```python
from build123d import *

# Parameters (mm, degrees)
ESQUISSE2_R = 0.5


with BuildPart() as part:
    # Balayage1: sweep along a path in Esquisse1
    with BuildLine(Plane.XY) as balayage1_path:
        Line((0, 0), (15, 0))
        ThreePointArc((15, 0), (17.492346414, 3.91220022), (12.893377781, 4.517665927))
        Line((12.893377781, 4.517665927), (11.143330468, 2.432040753))
        ThreePointArc((11.143330468, 2.432040753), (10.136256816, 1.85060651), (8.991054914, 2.052536503))
        Line((8.991054914, 2.052536503), (7.35, 3))
        ThreePointArc((7.35, 3), (6.5, 3.227756814), (5.65, 3))
        Line((5.65, 3), (3.35, 1.672094381))
        ThreePointArc((3.35, 1.672094381), (2.5, 1.444337567), (1.65, 1.672094381))
        Line((1.65, 1.672094381), (0, 2.624722325))
    # Esquisse2 → Balayage1 (sweep)
    with BuildSketch(Plane(origin=(0, 0, 0), x_dir=(0, 0, -1), z_dir=(1, 0, 0))):
        Circle(ESQUISSE2_R)
    sweep(path=balayage1_path.line)


solid = part.part
```
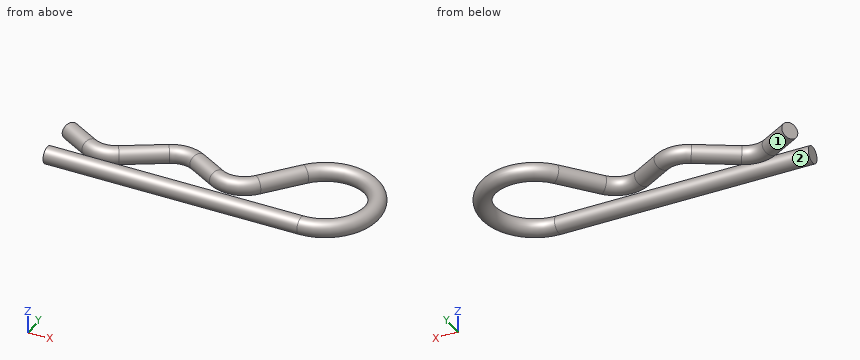
Input: part model. Units: mm. Frame: model coordinates. Face numbers are marked on the shaded views. A direction names the side the tool comes from. Round coordinates to 2 decimals unless told otherwise and drop trailing zeros. Order: outer loops, then holes, each group sorted by start corner. A loop starts at its lowest first (then second) coordinate and runs counter-clockwise, first axis right, second up. Notation, with made-up numbers: (-2.75, 47) - (13.25, 47) arc R24 cw to (13.25, 86) - close; hole circle Ø5 at (3, 84). An arc over 180 degrees is marked (long way). Answer in a Markdown table with one row per item.
Item 1: Line query: line 1 (Z direction, x = 12.5, y = 4); line 2 (Y direction, x = 14.5, z = -0.4); line 3 (Y direction, x = 6, z = 0). Output: solid intervals per line, ascending.
Model answer:
| item | result |
|---|---|
| line 1 | z = -0.5 to 0.5 |
| line 2 | y = -0.3 to 0.3, 5.15 to 5.76 |
| line 3 | y = -0.5 to 0.5, 2.62 to 3.67 |
Item 2: Pin query (flat end, axial travel): pin 1 (0.5 mm diameter, centred on y = 0, z = 0, fed in from -X). Return the tip coordinate at first contact, or that it passes through.
Model answer:
| item | result |
|---|---|
| pin 1 | stops at x = 0 |
Item 3: Reachability of the marked faces 1 and 2 from +Z, -Z, +X, -X, +Y, -Y: full face, straight path, thin tool, end or side. Return the list, or none.
Model answer:
| item | result |
|---|---|
| face 1 | none |
| face 2 | -X |
Item 4: Section query A-A (z = 0.15). Return the cut outline in (x, y), then the cut area to 3 significant figures.
Model answer:
| item | result |
|---|---|
| outline | (-0.24, 2.21) - (1.41, 1.26) arc R2.18 ccw to (3.59, 1.26) - (5.89, 2.59) arc R1.22 cw to (7.11, 2.59) - (8.75, 1.64) arc R2.18 ccw to (11.51, 2.13) - (13.26, 4.21) arc R2.27 cw (long way) to (15, 0.48) - (0, 0.48) - (0, -0.48) - (15, -0.48) arc R3.23 ccw (long way) to (12.53, 4.82) - (10.78, 2.74) arc R1.22 cw to (9.23, 2.47) - (7.59, 3.41) arc R2.18 ccw to (5.41, 3.41) - (3.11, 2.09) arc R1.22 cw to (1.89, 2.09) - (0.24, 3.04) - close |
| area | 39.3 mm² |
